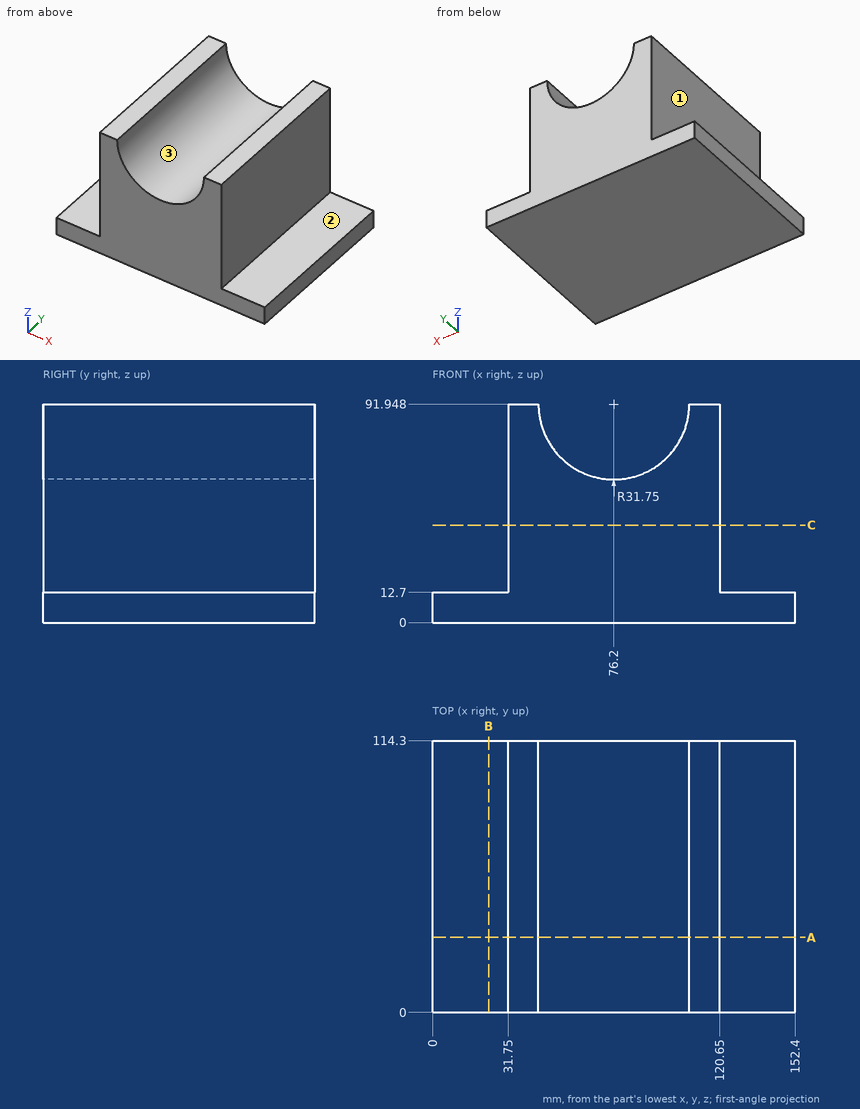
Can you work these out from the drawing? Everything is in mm from the part's minimum corner. A direction names the side the tool comes from. Coordinates: 2 decimals unless noted, no trailing zeros. Loops run counter-clockwise (first coordinate to the right, second up) from the corner with the lowest first, then second, coordinate; pieces in that order, holes last. Notation, with made-up numbers: (44, -29) - (59, -29) arc R27 ccw to (59, -5) - close; hole circle Ø10 at (52.25, -33). An arc over 180 degrees is marked (long way). Use a Markdown table: item, result.
Item 1: If I drill on probe 1 along X at (y, z) = (45.5, 51.5); probe 2 along Z at (x, y) = (18, 54); probe 3 along X at (y, z) = (33, 67.5), over which ranges is the centre line in solid material (lowest first)? Write a range as from..to.
Numbers:
| item | result |
|---|---|
| probe 1 | x = 31.75..120.65 |
| probe 2 | z = 0..12.7 |
| probe 3 | x = 31.75..55.94, 96.46..120.65 |
Item 2: I want a section at A-A on y = 31.5. Please give me the cut outline in (x, z), and give its area (3 significant figures).
Numbers:
| item | result |
|---|---|
| outline | (0, 0) - (152.4, 0) - (152.4, 12.7) - (120.65, 12.7) - (120.65, 91.95) - (107.95, 91.95) arc R31.75 cw to (44.45, 91.95) - (31.75, 91.95) - (31.75, 12.7) - (0, 12.7) - close |
| area | 7,400 mm2 |
Item 3: Will these pins go through, and if not, where does the flat tip stop? pin 1 (24 mm diameter, centred on y = 37.5, z = 60, fed in from -X); pin 2 (12 mm diameter, centred on x = 75, y = 35, fed in from +Z); pin 3 (9.5 mm diameter, centred on x = 16, y = 65.5, fed in from +Z).
Numbers:
| item | result |
|---|---|
| pin 1 | stops at x = 31.75 |
| pin 2 | stops at z = 61.03 |
| pin 3 | stops at z = 12.7 |
Item 4: For the marked faces 1, 2 and 3, which set-ups out of +Z, -Z, +X, -X, +Y, -Y let a thin tool reach every point of the face, with its end or its side?
Numbers:
| item | result |
|---|---|
| face 1 | +Z, -X, +Y, -Y |
| face 2 | +Z, +X, +Y, -Y |
| face 3 | +Z, +Y, -Y |
Item 5: I want a section at C-C on z = 41. Please give me the cut outline in (x, y).
Numbers:
| item | result |
|---|---|
| outline | (31.75, 0) - (120.65, 0) - (120.65, 114.3) - (31.75, 114.3) - close |
Item 6: I want a section at B-B on x = 23.5. Please give me the cut outline in (y, z), and give its area (3 significant figures).
Numbers:
| item | result |
|---|---|
| outline | (0, 0) - (114.3, 0) - (114.3, 12.7) - (0, 12.7) - close |
| area | 1,450 mm2 |
